from build123d import *

# Parameters (mm, degrees)
IZIM6_R               = 1.25
KES_EKSTR_ZYON1_DEPTH = 4


with BuildPart() as part:
    # Çizim5 → Döndür1 (revolve)
    with BuildSketch(Plane(origin=(0, 0, 0), x_dir=(1, 0, 0), z_dir=(0, 1, 0)), mode=Mode.PRIVATE) as d_nd_r1_sk:
        with BuildLine():
            Line((0, 0), (0, -2.45))
            Line((0, -2.45), (1, -2.9))
            Line((1, -2.9), (1, -2.45))
            Line((1, -2.45), (6.8, -2.45))
            Line((6.8, -2.45), (8.8, -6.2))
            Line((8.8, -6.2), (10.2, -6.2))
            Line((10.2, -6.2), (10.2, -3.2))
            Line((10.2, -3.2), (11.85, -3.2))
            ThreePointArc((11.85, -3.2), (17.6, -6.75), (23.35, -3.2))
            Line((23.35, -3.2), (25, -3.2))
            Line((25, -3.2), (25, -6.75))
            Line((25, -6.75), (27.8, -6.75))
            Line((27.8, -6.75), (27.8, 0))
            Line((27.8, 0), (0, 0))
        make_face()
    revolve(d_nd_r1_sk.sketch.rotate(Axis((27.8, 0, 0), (-1, 0, 0)), 180), axis=Axis((27.8, 0, 0), (-1, 0, 0)))

    # Çizim6 → Kes-Ekstrüzyon1 (cut)
    with BuildSketch(Plane.ZY):
        Circle(IZIM6_R)
    extrude(amount=-KES_EKSTR_ZYON1_DEPTH, mode=Mode.SUBTRACT)


solid = part.part
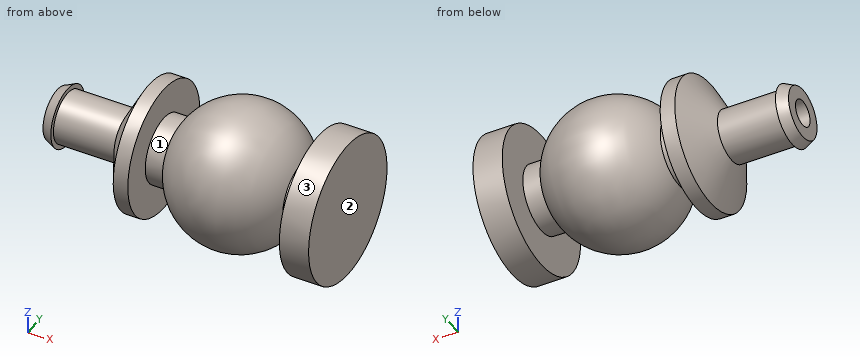
Source: CAD feature listing. Evaluate the final solid. Frame: model axes, mm. Face numbers are marked on the shaded views. Give positions to 0.01 mm unless a question says otherwise; leave off trailing zeros. Write each loop counter-clockwise with the first axis right and the second up, starting at its lowest first coordinate (ties: lowest second). Pieces come first, ordered by that corner, then holes. Notation, with made-up numbers: M -37,31 L -31,31 A20 ccw -31,62 Z; hole C 46,54.25 d4. An arc over 180 degrees is marked long. Return JSON: item names as keys, results as strings. Group by question number.
1) Cut plane B-B, the plane y = -4.75. Give the number of separate pieces and of enclosed holes in the cut face, plus the area to 3 significant figures.
2) Pull-direction query (X, two-part tool) for the marked faces 1, 2 and 3; classes: pulls with the +X half, pulls with the -X half, needs draft (parallel to the pull), parting line crosses it, or undercut.
3) Pin query (flat end, axial travel): P1, Ø1.5, axis at x = 6, y = 4.5, coming from the +Z side; P2, Ø3, axis at y = 2.5, z = 4.5, coming from the -X side; P3, Ø2, axis at x = 21.5, y = 1.5, coming from the +Z side; P4, Ø3, axis at x = 4.5, y = 3.5, coming from the -Z side. Return the tip coordinate at first contact, or that it passes through.
4) Cut plane A-A, the plane x = 24. Output: boundary loops of the cut face in (y, z), plus the area to 3 significant figures.
5) Cut plane D-D, the plane x = 9.5. Output: boundary loops of the cut face in (y, z).
6) Material intervals for line 1 along X through (y, z) = (5, -1); line 2 along Y through (x, z) = (1.7, 0); line 3 along X through (y, z) = (3.5, -1.5), sorted ascending. Write a range as [from, to].
Recorded:
{
 "1": {"separate pieces": "3", "enclosed holes": "0", "area": "112 mm²"},
 "2": {"face 1": "undercut", "face 2": "pulls with the +X half", "face 3": "needs draft"},
 "3": {"P1": "passes through", "P2": "stops at x = 7.44", "P3": "stops at z = 5.92", "P4": "stops at z = -1.42"},
 "4": {"outline": "C 0,0 d6.4", "area": "32.2 mm²"},
 "5": {"outline": "C 0,0 d12.4"},
 "6": {"line 1": "x = [8.21, 10.2], [13.3, 21.9], [25, 27.8]", "line 2": "y = [-2.45, -1.25], [1.25, 2.45]", "line 3": "x = [7.52, 10.2], [12.2, 23], [25, 27.8]"}
}
